```python
from build123d import *

# Parameters (mm, degrees)
CROQUIS1_R              = 11.5
CROQUIS1_W              = 20
CROQUIS1_H              = 67.5
CROQUIS1_W_2            = 27
CROQUIS1_H_2            = 14
SALIENTE_EXTRUIR1_DEPTH = 3
CROQUIS2_R              = 2.5
CROQUIS2_R_2            = 1.5
CORTAR_EXTRUIR1_DEPTH   = 4
REDONDEO1_R             = 3
CROQUIS3_R              = 0.75
CORTAR_EXTRUIR2_DEPTH   = 4
CROQUIS4_W              = 8
CROQUIS4_H              = 3
SALIENTE_EXTRUIR2_DEPTH = 3


with BuildPart() as part:
    # Croquis1 → Saliente-Extruir1 (new body)
    with BuildSketch(Plane.XY):
        Circle(CROQUIS1_R)
        with Locations((0, -33.75)):
            Rectangle(CROQUIS1_W, CROQUIS1_H)
        with Locations((0, -74.5)):
            Rectangle(CROQUIS1_W_2, CROQUIS1_H_2)
    extrude(amount=SALIENTE_EXTRUIR1_DEPTH)

    # Croquis2 → Cortar-Extruir1 (cut, through all)
    with BuildSketch(Plane.XY.offset(3)):
        Circle(CROQUIS2_R)
        with Locations((0, -31.5)):
            Circle(CROQUIS2_R_2)
        with Locations((0, -67.5)):
            Circle(CROQUIS2_R_2)
    extrude(amount=-CORTAR_EXTRUIR1_DEPTH, mode=Mode.SUBTRACT)

    # Redondeo1
    redondeo1_edges = [part.edges().sort_by_distance(p)[0] for p in [
        (13.5, -67.5, 1.5),
        (-13.5, -67.5, 1.5),
    ]]
    fillet(redondeo1_edges, radius=REDONDEO1_R)

    # Croquis3 → Cortar-Extruir2 (cut, through all)
    with BuildSketch(Plane.XY.offset(3)):
        with Locations((0, -16)):
            Circle(CROQUIS3_R)
        with Locations((0, 8)):
            Circle(CROQUIS3_R)
    extrude(amount=-CORTAR_EXTRUIR2_DEPTH, mode=Mode.SUBTRACT)

    # Croquis4 → Saliente-Extruir2 (add)
    with BuildSketch(Plane.XY.offset(3)):
        with Locations((-6.5, -83)):
            Rectangle(CROQUIS4_W, CROQUIS4_H)
        with Locations((6.5, -83)):
            Rectangle(CROQUIS4_W, CROQUIS4_H)
    extrude(amount=-SALIENTE_EXTRUIR2_DEPTH)


solid = part.part
```
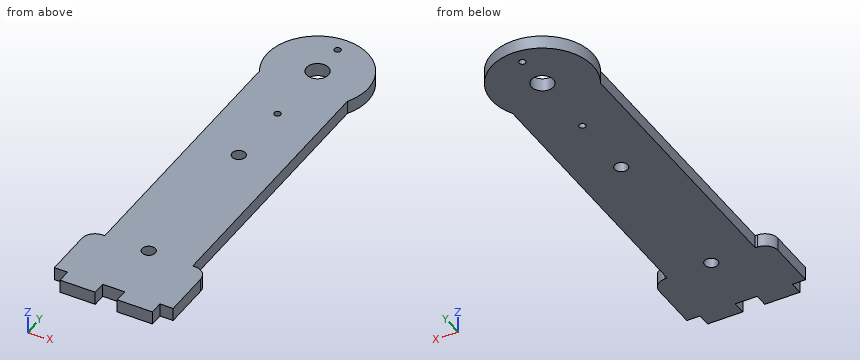
For this review, take the finished solid that the model builds, in its own axes (mm). Coordinates: 2 decimals unless noted, no trailing zeros. Write each loop counter-clockwise with the first axis right and the second up, starting at its lowest first coordinate (ties: lowest second). Pieces come first, ordered by that corner, then holes. Notation, with made-up numbers: (-31.5, 64) - (18.5, 64) arc R10 cw to (18.5, 69) - close; hole circle Ø6 at (-27.5, 63). An arc over 180 degrees is marked (long way). Answer in a Markdown table with one row per item. Add a question column.
Q1. For probe 1 along X at (y, z) = (-35.5, 0.8); probe 2 along Y at (x, z) = (2, 2.8); probe 3 along Y at (x, z) = (2.25, 2.75), list the stretches that pass through material, from the lowest coordinate up.
Q2. We need section B-B, the plane y = 0. State the section outline as (x, z) points.
Q3. We need section A-A, the plane z = 1.75. State the section outline as (x, y) points.
Q4. We need section C-C, the plane y = -31.5. State the section outline as (x, z) points.
Q5. We need section D-D, the plane y = -51.5. State the section outline as (x, z) points, and give its area (3 significant figures).
Q6. For P1, Ø1.5, axis at y = -83, z = 2, coming from the -X side; P2, Ø0.6, axis at x = 10, z = 2, coming from the +Y side; P3, Ø1.5, axis at x = 12, z = 1.5, coming from the -Y side, all flat-tipped, find the tip position at first contact; note any pin that passes through.
Answer list:
| question | item | result |
|---|---|---|
| 1 | probe 1 | x = -10 to 10 |
| 1 | probe 2 | y = -81.5 to -1.5, 1.5 to 11.32 |
| 1 | probe 3 | y = -81.5 to -1.09, 1.09 to 11.28 |
| 2 | outline | (-11.5, 0) - (-2.5, 0) - (-2.5, 3) - (-11.5, 3) - close; (2.5, 0) - (11.5, 0) - (11.5, 3) - (2.5, 3) - close |
| 3 | outline | (-13.5, -81.5) - (-10.5, -81.5) - (-10.5, -84.5) - (-2.5, -84.5) - (-2.5, -81.5) - (2.5, -81.5) - (2.5, -84.5) - (10.5, -84.5) - (10.5, -81.5) - (13.5, -81.5) - (13.5, -70.5) arc R3 ccw to (10.5, -67.5) - (10, -67.5) - (10, -5.68) arc R11.5 ccw (long way) to (-10, -5.68) - (-10, -67.5) - (-10.5, -67.5) arc R3 ccw to (-13.5, -70.5) - close; hole circle Ø5 at (0, 0); hole circle Ø3 at (0, -67.5); hole circle Ø3 at (0, -31.5); hole circle Ø1.5 at (0, -16); hole circle Ø1.5 at (0, 8) |
| 4 | outline | (-10, 0) - (-1.5, 0) - (-1.5, 3) - (-10, 3) - close; (1.5, 0) - (10, 0) - (10, 3) - (1.5, 3) - close |
| 5 | outline | (-10, 0) - (10, 0) - (10, 3) - (-10, 3) - close |
| 5 | area | 60.0 mm2 |
| 6 | P1 | stops at x = -10.5 |
| 6 | P2 | stops at y = 6.18 |
| 6 | P3 | stops at y = -81.5 |
